Here's how the part is built. I have some questions about the finished solid (model axes, mm). Face numbers are marked on the shaded views. A direction names the side the tool comes from. Round coordinates to 2 decimals unless told otherwise and drop trailing zeros. Order: outer loops, then holes, each group sorted by start corner. A loop starts at its lowest first (then second) coordinate and runs counter-clockwise, first axis right, second up. Notation, with made-up numbers: (9, 27.25) -> (59, 27.25) arc R29 cw to (59, 64.25) -> close; hole circle Ø9 at (-3.5, 59). An arc over 180 degrees is marked (long way). Use a Markdown table: item, result. Add a question column.
(1) I'm going to push flat-ended pins straight in: P1, Ø8, axis at x = 7, y = 5.5, coming from the -Z side; P2, Ø4.5, axis at y = 6.5, z = -46, coming from the -X side; P3, Ø14, axis at x = -24.5, z = -61.5, coming from the +Y side; P4, Ø2.5, axis at x = 0, z = -2.75, coming from the -Y side. Where does each tip first touch, or does it pass through?
(2) I want a section at D-D, the plane z = -44. Please give me the cut outline in (x, y).
(3) If I drill on probe 1 along Y at (x, z) = (-5, -54.5); probe 2 along Y at (x, z) = (-10, -19); probe 3 along X at (y, z) = (1.25, -6.5), over which ranges is the centre line in solid material (lowest first)?
(4) Thinking about a two-plate mould opening in Z: for the marked faces 4 and 5, which applies, pulls with the +Z half, pulls with the -Z half, needs draft (parallel to the pull), parting line crosses it, or undercut?
(5) I want a section at C-C, the plane z = -58.5. Please give me the cut outline in (x, y).
(6) I want a section at A-A, the plane y = 5. Please give me the cut outline in (x, z).
(7) On a 3-axis mill with a long thin cutter (end or side, diameter ignored), from which of +Z, -Z, +X, -X, +Y, -Y can I reach the whole of each face in a straight line? I mean the marked faces 1, 2 and 3. Say none if no direction works.
(8) I want a section at B-B, the plane z = -28.7. Please give me the cut outline in (x, y), then the cut area to 3 significant figures.
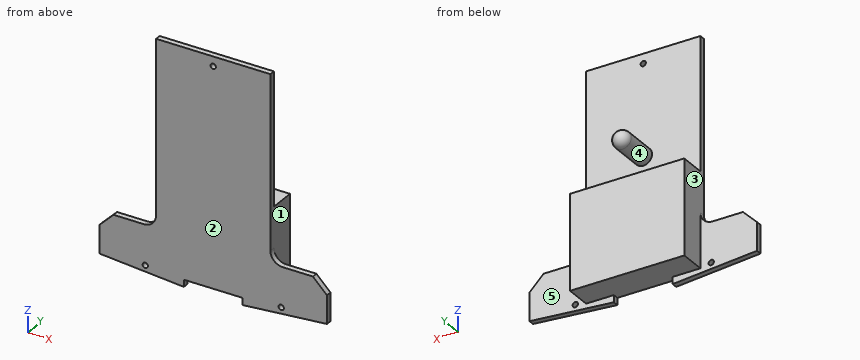
from build123d import *

# Parameters (mm, degrees)
SKETCH1_R           = 0.75
BOSS_EXTRUDE1_DEPTH = 1.6
SKETCH2_W           = 32.5
SKETCH2_H           = 27
BOSS_EXTRUDE2_DEPTH = 7.35
SKETCH3_R           = 2.5
BOSS_EXTRUDE3_DEPTH = 12
FILLET1_R           = 2.5


with BuildPart() as part:
    # Sketch1 → Boss-Extrude1 (new body)
    with BuildSketch(Plane(origin=(0, 0, 0), x_dir=(1, 0, 0), z_dir=(0, 1, 0))):
        with BuildLine():
            Line((-16.25, 0), (16.25, 0))
            Line((16.25, 0), (16.25, 49.14))
            ThreePointArc((16.25, 49.14), (17.275126266, 51.614873734), (19.75, 52.64))
            Line((19.75, 52.64), (28.35, 52.64))
            Line((28.35, 52.64), (32.35, 56.64))
            Line((32.35, 56.64), (32.35, 64.64))
            Line((32.35, 64.64), (8.35, 66.64))
            Line((8.35, 66.64), (8.35, 64.64))
            Line((8.35, 64.64), (-8.35, 64.64))
            Line((-8.35, 64.64), (-8.35, 66.64))
            Line((-8.35, 66.64), (-32.35, 64.64))
            Line((-32.35, 64.64), (-32.35, 56.64))
            Line((-32.35, 56.64), (-28.35, 52.64))
            Line((-28.35, 52.64), (-19.75, 52.64))
            ThreePointArc((-19.75, 52.64), (-17.275126266, 51.614873734), (-16.25, 49.14))
            Line((-16.25, 49.14), (-16.25, 0))
        make_face()
        with Locations(Location((-19.33, 63.968934124, 0), (0, 0, 270))):
            Circle(SKETCH1_R, mode=Mode.SUBTRACT)
        with Locations(Location((19.33, 63.968934124, 0), (0, 0, 270))):
            Circle(SKETCH1_R, mode=Mode.SUBTRACT)
        with Locations(Location((0, 2.75, 0), (0, 0, 270))):
            Circle(SKETCH1_R, mode=Mode.SUBTRACT)
    extrude(amount=BOSS_EXTRUDE1_DEPTH)

    # Sketch2 → Boss-Extrude2 (add)
    with BuildSketch(Plane(origin=(0, 1.6, 0), x_dir=(1, 0, 0), z_dir=(0, 1, 0))):
        with Locations((0, 51.14)):
            Rectangle(SKETCH2_W, SKETCH2_H)
    extrude(amount=BOSS_EXTRUDE2_DEPTH)

    # Sketch3 → Boss-Extrude3 (add)
    with BuildSketch(Plane(origin=(0, 1.6, 0), x_dir=(1, 0, 0), z_dir=(0, 1, 0))):
        with Locations(Location((0, 28.7, 0), (0, 0, 90))):
            Circle(SKETCH3_R)
    extrude(amount=BOSS_EXTRUDE3_DEPTH)

    # Fillet1
    fillet1_edges = [part.edges().sort_by_distance(p)[0] for p in [
        (0, 13.6, -26.2),
    ]]
    fillet(fillet1_edges, radius=FILLET1_R)


solid = part.part
Taken from the geometry:
| question | item | result |
|---|---|---|
| 1 | P1 | stops at z = -64.64 |
| 1 | P2 | stops at x = -16.25 |
| 1 | P3 | stops at y = 1.6 |
| 1 | P4 | stops at y = 0 |
| 2 | outline | (-16.25, 0) -> (16.25, 0) -> (16.25, 8.95) -> (-16.25, 8.95) -> close |
| 3 | probe 1 | y = 0 to 8.95 |
| 3 | probe 2 | y = 0 to 1.6 |
| 3 | probe 3 | x = -16.25 to 16.25 |
| 4 | face 4 | undercut |
| 4 | face 5 | needs draft |
| 5 | outline | (-32.35, 0) -> (32.35, 0) -> (32.35, 1.6) -> (16.25, 1.6) -> (16.25, 8.95) -> (-16.25, 8.95) -> (-16.25, 1.6) -> (-32.35, 1.6) -> close |
| 6 | outline | (-16.25, -64.64) -> (16.25, -64.64) -> (16.25, -37.64) -> (-16.25, -37.64) -> close; circle Ø5 at (0, -28.7) |
| 7 | face 1 | +Z, +X, +Y |
| 7 | face 2 | +Z, -Z, +X, -X, -Y |
| 7 | face 3 | +Z, -X, +Y |
| 8 | outline | (-16.25, 0) -> (16.25, 0) -> (16.25, 1.6) -> (2.5, 1.6) -> (2.5, 11.1) arc R2.5 ccw to (-2.5, 11.1) -> (-2.5, 1.6) -> (-16.25, 1.6) -> close |
| 8 | area | 109 mm2 |
